Input: part model. Units: mm. Frame: model coordinates. Face numbers are marked on the shaded views. A direction names the side the tool comes from. Give positions to 0.01 mm unless a question says otherwise; leave off trailing zeros. Loops run counter-clockwise (first coordinate to the right, second up) from the corner with the lowest first, then second, coordinate; pieces in that order, holes last. Notation, with made-up numbers: (34.5, 88) -> (86.5, 88) arc R13 ccw to (86.5, 95) -> close; hole circle Ø11 at (-27, 35). An arc over 180 degrees is marked (long way). Answer in a Markdown table with one row per item. Add a question column.
```python
from build123d import *

# Parameters (mm, degrees)
SKETCH1_R           = 11.15
SKETCH1_R_2         = 1.7
BOSS_EXTRUDE1_DEPTH = 8
BOSS_EXTRUDE2_START = 3
SKETCH2_R           = 4.5
SKETCH2_R_2         = 1.7
BOSS_EXTRUDE2_DEPTH = 3


with BuildPart() as part:
    # Sketch1 → Boss-Extrude1 (new body)
    with BuildSketch(Plane.XY):
        with BuildLine():
            Line((65, 1.454102171), (65, 35))
            Line((65, 35), (55.375185128, 64.942285128))
            ThreePointArc((55.375185128, 64.942285128), (42.229542157, 75.995363133), (26.562387746, 68.958408169))
            Line((26.562387746, 68.958408169), (-13.437612254, 8.958408169))
            ThreePointArc((-13.437612254, 8.958408169), (-13.067754119, -9.489799908), (4.360524021, -15.550187467))
            Line((4.360524021, -15.550187467), (65, 1.454102171))
        make_face()
        Circle(SKETCH1_R, mode=Mode.SUBTRACT)
        with Locations((57.5, 24.966666667)):
            Circle(SKETCH1_R_2, mode=Mode.SUBTRACT)
        with Locations((57.5, 10.033333333)):
            Circle(SKETCH1_R_2, mode=Mode.SUBTRACT)
        with Locations((40, 60)):
            Circle(SKETCH1_R, mode=Mode.SUBTRACT)
    extrude(amount=-BOSS_EXTRUDE1_DEPTH)

    # Sketch2 → Boss-Extrude2 (add)
    with BuildSketch(Plane.XY.offset(BOSS_EXTRUDE2_START)):
        with BuildLine():
            Line((4.360524021, -15.550187467), (65, 1.454102171))
            Line((65, 1.454102171), (65, 35))
            Line((65, 35), (55.375185128, 64.942285128))
            ThreePointArc((55.375185128, 64.942285128), (42.229542157, 75.995363133), (26.562387746, 68.958408169))
            Line((26.562387746, 68.958408169), (-13.437612254, 8.958408169))
            ThreePointArc((-13.437612254, 8.958408169), (-13.067754119, -9.489799908), (4.360524021, -15.550187467))
        make_face()
        Circle(SKETCH2_R, mode=Mode.SUBTRACT)
        with Locations((57.5, 24.966666667)):
            Circle(SKETCH2_R_2, mode=Mode.SUBTRACT)
        with Locations((57.5, 10.033333333)):
            Circle(SKETCH2_R_2, mode=Mode.SUBTRACT)
        with Locations((40, 60)):
            Circle(SKETCH2_R, mode=Mode.SUBTRACT)
    extrude(amount=-BOSS_EXTRUDE2_DEPTH)


solid = part.part
```
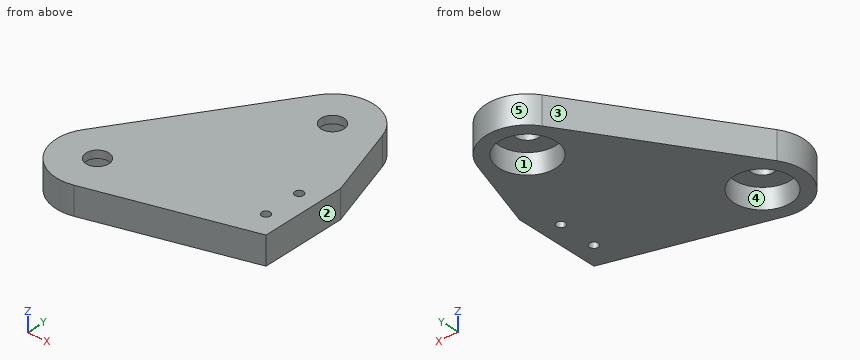
1) Section B-B on z = -7. Output: boundary loops of the cut face in (x, y), and give its area (3 significant figures).
2) Pin query (flat end, axial travel): pin 1 (5 mm diameter, centred on y = -6, z = -3, fed in from -X); pin 2 (5 mm diameter, centred on y = 63.5, z = -5, fed in from +X); pin 3 (10.5 mm diameter, centred on x = 0, y = 0, fed in from -Z). Return the tip coordinate at first contact, or that it passes through.
3) Section D-D on x = 57.5. Output: boundary loops of the cut face in (y, z), and give its area (3 significant figures).
4) Section A-A on y = -1. Output: boundary loops of the cut face in (x, z), and give its area (3 significant figures).
5) Reachability of the marked faces 4 and 5 from +Z, -Z, +X, -X, +Y, -Y: full face, straight path, thin tool, end or side. Return the list, or none.
6) Pull-direction query (Y, two-part tool) for the marked faces 1, 2 and 3; classes: +Y half, -Y half, draft (parallel to the pull), parting line (faces both ways), or undercut.
7) Section C-C on x = 0. Output: boundary loops of the cut face in (y, z).
8) Material intervals for line 1 along Z through (x, y) = (33, 67.5); line 2 along Y through (x, z) = (-3, -4.5); line 3 along X through (y, z) = (64.5, -3.75), sorted ascending.
Working result:
| question | item | result |
|---|---|---|
| 1 | outline | (-13.44, 8.96) arc R16.15 ccw to (4.36, -15.55) -> (65, 1.45) -> (65, 35) -> (55.38, 64.94) arc R16.15 ccw to (26.56, 68.96) -> close; hole circle Ø22.3 at (0, 0); hole circle Ø22.3 at (40, 60); hole circle Ø3.4 at (57.5, 10.03); hole circle Ø3.4 at (57.5, 24.97) |
| 1 | area | 4,080 mm2 |
| 2 | pin 1 | stops at x = -15.77 |
| 2 | pin 2 | stops at x = 56.64 |
| 2 | pin 3 | stops at z = 0 |
| 3 | outline | (-0.65, -8) -> (8.33, -8) -> (8.33, 3) -> (-0.65, 3) -> close; (11.73, -8) -> (23.27, -8) -> (23.27, 3) -> (11.73, 3) -> close; (26.67, -8) -> (58.33, -8) -> (58.33, 3) -> (26.67, 3) -> close |
| 3 | area | 574 mm2 |
| 4 | outline | (-16.12, -8) -> (-11.11, -8) -> (-11.11, 0) -> (-4.39, 0) -> (-4.39, 3) -> (-16.12, 3) -> close; (4.39, 0) -> (11.11, 0) -> (11.11, -8) -> (56.25, -8) -> (56.25, 3) -> (4.39, 3) -> close |
| 4 | area | 592 mm2 |
| 5 | face 4 | -Z |
| 5 | face 5 | +Z, -Z, +Y |
| 6 | face 1 | undercut |
| 6 | face 2 | draft |
| 6 | face 3 | +Y half |
| 7 | outline | (-16.15, -8) -> (-11.15, -8) -> (-11.15, 0) -> (-4.5, 0) -> (-4.5, 3) -> (-16.15, 3) -> close; (4.5, 0) -> (11.15, 0) -> (11.15, -8) -> (29.11, -8) -> (29.11, 3) -> (4.5, 3) -> close |
| 8 | line 1 | z = 0 to 3 |
| 8 | line 2 | y = -15.87 to -10.74, 10.74 to 24.61 |
| 8 | line 3 | x = 23.59 to 29.8, 50.2 to 55.52 |
